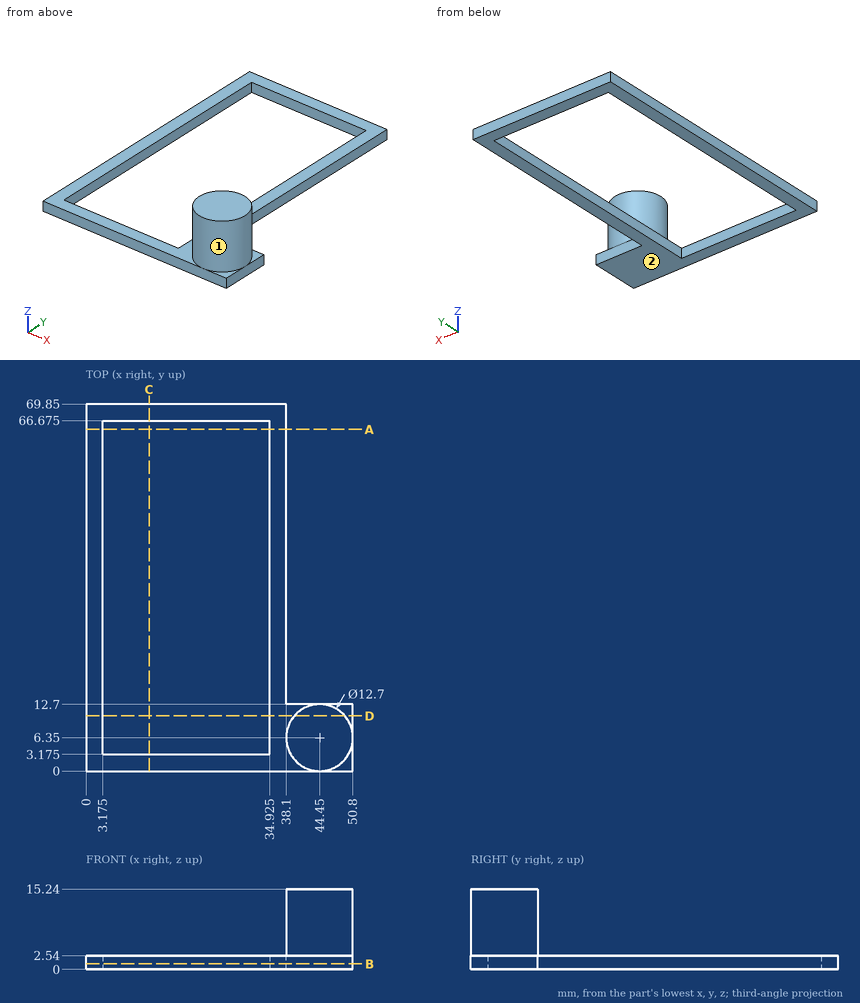
Job drawing, mm, ordinate dimensions from the low corner. One solid piece. A direction names the side the tool comes from. Round coordinates to 2 decimals unless told otherwise and drop trailing zeros. Loops run counter-clockwise (first coordinate to the right, second up) from the corner with the lowest first, then second, coordinate; pieces in that order, holes last. Notation, with made-up numbers: (-31, 4.5) -> (14, 4.5) arc R30 cw to (14, 40.5) -> close; hole circle Ø5 at (36.25, 57.5). An arc over 180 degrees is marked (long way). One line per item, written item: value. Start each with the question number.
Q1. Cut at B-B on z = 1. List the corners of the cut face in (x, y) (3 decimals), plus the area to 3 significant figures.
Q2. 3-axis set-ups, long thin cutter, end or side, ignore diameter. For the marked faces 1 and 2: which of +Z, -Z, +X, -X, +Y, -Y reach the whole face in a straight line?
Q3. Drop flat-ended pins along their axis: pin 1 Ø3 at (x, z) = (41.5, 1.5) entering from +Y; pin 2 Ø8 at (x, y) = (40.5, 30.5) entering from +Z; pin 3 Ø0.8 at (y, z) = (33, 1.5) entering from +X; pin 4 Ø2 at (y, z) = (29.5, 1.5) entering from -X. Give the stop position or say it passes through.
Q4. Cut at C-C on x = 12. List the corners of the cut face in (y, z) (3 decimals), plus the area to 3 significant figures.
Q5. Cut at D-D on y = 10.5. List the corners of the cut face in (x, z) (3 decimals), plus the area to 3 significant figures.
Q6. Probe line 1 along X through (y, z) = (33, 2) (3 decimals); line 2 along X through (y, z) = (11, 2.25) (3 decimals); line 3 along X through (y, z) = (6, 9.25). List the from-to ranges inside material, lowest first.
Q7. Cut at A-A on y = 65. List the corners of the cut face in (x, z) (3 decimals), plus the area to 3 significant figures.
Computed:
1. outline: (0, 0) -> (50.8, 0) -> (50.8, 12.7) -> (38.1, 12.7) -> (38.1, 69.85) -> (0, 69.85) -> close; hole (3.175, 3.175) -> (34.925, 3.175) -> (34.925, 66.675) -> (3.175, 66.675) -> close
1. area: 806 mm²
2. face 1: +Z
2. face 2: -Z, +X, -X, +Y, -Y
3. pin 1: y = 12.7
3. pin 2: z = 2.54
3. pin 3: x = 38.1
3. pin 4: x = 0
4. outline: (0, 0) -> (3.175, 0) -> (3.175, 2.54) -> (0, 2.54) -> close; (66.675, 0) -> (69.85, 0) -> (69.85, 2.54) -> (66.675, 2.54) -> close
4. area: 16.1 mm²
5. outline: (0, 0) -> (3.175, 0) -> (3.175, 2.54) -> (0, 2.54) -> close; (34.925, 0) -> (50.8, 0) -> (50.8, 2.54) -> (49.256, 2.54) -> (49.256, 15.24) -> (39.644, 15.24) -> (39.644, 2.54) -> (34.925, 2.54) -> close
5. area: 170 mm²
6. line 1: 0 to 3.175, 34.925 to 38.1
6. line 2: 0 to 3.175, 34.925 to 50.8
6. line 3: 38.11 to 50.79
7. outline: (0, 0) -> (3.175, 0) -> (3.175, 2.54) -> (0, 2.54) -> close; (34.925, 0) -> (38.1, 0) -> (38.1, 2.54) -> (34.925, 2.54) -> close
7. area: 16.1 mm²
